```python
from build123d import *

# Parameters (mm, degrees)
F0_W     = 98.4343141317
F0_H     = 49.9388501048
F1_DEPTH = 152.4
F3_DEPTH = 25.4
F4_DEPTH = 101.6
F6_D     = 25.4


with BuildPart() as f1:
    # F0 (on Front) → F1 (new body)
    with BuildSketch(Plane.XZ):
        with Locations((49.2171570659, -24.9694250524)):
            Rectangle(F0_W, F0_H)
    extrude(amount=F1_DEPTH)

    # F2 (on face) → F3 (join)
    with BuildSketch(Plane(origin=(0, 0, -49.9388501048), x_dir=(1, 0, 0), z_dir=(0, 0, -1))):
        with BuildLine():
            ThreePointArc((49.4931302965, 152.4), (82.2706467442, 139.9142220829), (98.4343141317, 108.7855200338))
            Line((98.4343141317, 108.7855200338), (98.4343141317, 152.4))
            Line((98.4343141317, 152.4), (49.4931302965, 152.4))
        make_face()
    extrude(amount=F3_DEPTH)

    # F4 (cut): a face of the model
    f4_faces = [f1.faces().sort_by_distance(p)[0] for p in [
        (87.4379245135, -141.7394263284, -75.3388501048),
    ]]
    extrude(f4_faces, amount=-F4_DEPTH, mode=Mode.SUBTRACT)

    # F6 (through all)
    with Locations(Plane(origin=(0, 0, -49.9388501048), x_dir=(1, 0, 0), z_dir=(0, 0, -1))):
        with Locations((57.5145594776, 113.6788129807)):
            Hole(F6_D / 2)


solid = f1.part
```
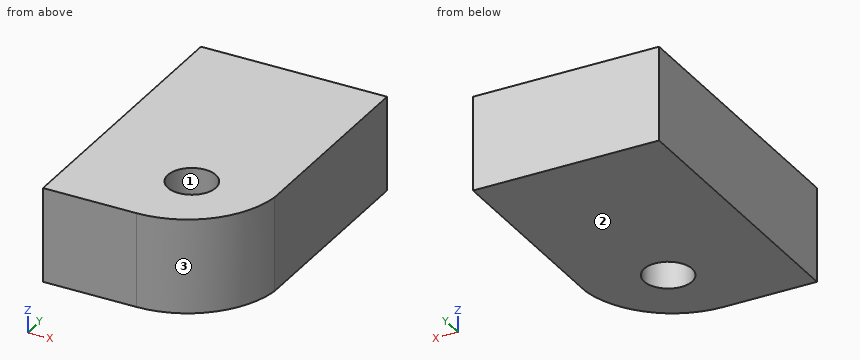
Design review of the part built by this model. Coordinates are the model's own, in mm. Face numbers are marked on the shaded views. Give positions to 0.01 mm unless a question says otherwise; leave off trailing zeros. Loops run counter-clockwise (first coordinate to the right, second up) from the corner with the lowest first, then second, coordinate; pieces in that order, holes last. Notation, with made-up numbers: (59, -35.75) -> (112, -35.75) arc R15 cw to (112, -12.75) -> close; hole circle Ø11 at (65.5, 80). An arc over 180 degrees is marked (long way). One line per item, written item: value.
Q1. We need section C-C on z = -2.5. Give the boundary of the cut face in (x, y).
Numbers:
outline: (0, -152.4) -> (49.49, -152.4) arc R49.27 ccw to (98.43, -108.79) -> (98.43, 0) -> (0, 0) -> close; hole circle Ø25.4 at (57.51, -113.68)
Q2. We need section D-D on x = 88.5. Give the boundary of the cut face in (y, z), and give its area (3 significant figures).
Numbers:
outline: (-133.23, -49.94) -> (0, -49.94) -> (0, 0) -> (-133.23, 0) -> close
area: 6,650 mm^2
Q3. We need section B-B on y = -107. Give the boundary of the cut face in (x, z).
Numbers:
outline: (0, -49.94) -> (46.71, -49.94) -> (46.71, 0) -> (0, 0) -> close; (68.32, -49.94) -> (98.43, -49.94) -> (98.43, 0) -> (68.32, 0) -> close
Q4. For pin 1 Ø2 at (x, y) = (68.5, -115.5) entering from -Z; pin 2 Ø1 at (y, z) = (-119.5, -29.5) entering from +X; pin 3 Ø10 at (x, z) = (70, -33.5) entering from -Y, all flat-tipped, find the tip position at first contact; note any pin that passes through.
Numbers:
pin 1: passes through
pin 2: stops at x = 96.13
pin 3: stops at y = -149.9
Q5. For L1, parallel to Y at x = 69, z = -20; L2, parallel to Y at x = 50, z = -4.5; L3, parallel to Y at x = 74.5, z = -18.5, list the stretches that pass through material, from the lowest coordinate up.
Numbers:
L1: y = -148.37 to -119.1, -108.26 to 0
L2: y = -152.4 to -123.92, -103.44 to 0
L3: y = -145.58 to 0
Q6. Draft analysis for pull direction X (two halves, no side actions). For the marked faces 1, 2 and 3, state which applies: pulls with the +X half, pulls with the -X half, needs draft (parallel to the pull), parting line crosses it, or undercut.
Numbers:
face 1: undercut
face 2: needs draft
face 3: pulls with the +X half
Q7. We need section A-A on x = 67.5. Give the boundary of the cut face in (y, z), and give its area (3 significant figures).
Numbers:
outline: (-148.99, -49.94) -> (-121.53, -49.94) -> (-121.53, 0) -> (-148.99, 0) -> close; (-105.83, -49.94) -> (0, -49.94) -> (0, 0) -> (-105.83, 0) -> close
area: 6,660 mm^2
